Geometry check sheet. Reference: the model listing, model coordinates, mm. Give positions to 0.01 mm unless a question says otherwise; leave off trailing zeros. Write each loop counter-clockwise with the first axis right and the second up, starting at its lowest first coordinate (ties: lowest second). Pieces come first, ordered by that corner, then holes.
(1) Depth check by flat-ended pin: P1, Ø1.5, axis at y = -2, z = 54, coming from the +X side; P2, Ø3.5, axis at x = 52, z = 80, coming from the +Y side; P3, Ø2, axis at y = -1, z = 42.5, coming from the -X side; P4, Ø1.5, axis at x = -162, y = -3.5, coming from the +Z side. Enter the tip coordinate at first touch or a pass-through.
(2) Cross-section at A-A (y = -3.8). Count the separate pieces of the cut face and the enclosed holes in it, and give its area (3 significant figures).
(3) Thickness scan on line 1 along Z through (x, y) = (10, -2); line 2 along X through (y, z) = (-2.6, -29.5); line 3 along Z through (x, y) = (-170, -3.3). Record the ranges inside material, lowest first.
(4) Cross-section at C-C (x = -126.5). Record the boundary of the cut face in (y, z), and give its area (3 significant figures).
(5) Cross-section at B-B (z = 54.5). Record the boundary of the cut face in (x, y), and give its area (3 significant figures).
```python
from build123d import *

# Parameters (mm, degrees)
F0_R     = 3
F1_DEPTH = 5


with BuildPart() as f1:
    # F0 (on Front) → F1 (new body)
    with BuildSketch(Plane.XZ):
        Polygon((62, 118), (0, 118), (0, 0), (-278, 0), (-278, 20), (-338, 20), (-338, 0), (-378, 0), (-378, -62), (92, -62), (92, 0), (62, 0), align=None)
        with Locations((-368, -30)):
            Circle(F0_R, mode=Mode.SUBTRACT)
        with Locations((-170, -52)):
            Circle(F0_R, mode=Mode.SUBTRACT)
        with Locations((-328, 10)):
            Circle(F0_R, mode=Mode.SUBTRACT)
        with Locations((-288, 10)):
            Circle(F0_R, mode=Mode.SUBTRACT)
        with Locations((-170, -10)):
            Circle(F0_R, mode=Mode.SUBTRACT)
        with Locations((72, -30)):
            Circle(F0_R, mode=Mode.SUBTRACT)
        with Locations((10, 0)):
            Circle(F0_R, mode=Mode.SUBTRACT)
        with Locations((52, 0)):
            Circle(F0_R, mode=Mode.SUBTRACT)
        with Locations((10, 80)):
            Circle(F0_R, mode=Mode.SUBTRACT)
        with Locations((52, 80)):
            Circle(F0_R, mode=Mode.SUBTRACT)
    extrude(amount=F1_DEPTH)


solid = f1.part
```
Reply:
1. P1: stops at x = 62
1. P2: passes through
1. P3: stops at x = 0
1. P4: stops at z = 0
2. separate pieces: 1
2. enclosed holes: 10
2. area: 37,400 mm2
3. line 1: z = -62 to -3, 3 to 77, 83 to 118
3. line 2: x = -378 to -370.96, -365.04 to 69.04, 74.96 to 92
3. line 3: z = -62 to -55, -49 to -13, -7 to 0
4. outline: (-5, -62) - (0, -62) - (0, 0) - (-5, 0) - close
4. area: 310 mm2
5. outline: (0, -5) - (62, -5) - (62, 0) - (0, 0) - close
5. area: 310 mm2
